Input: dimensioned drawing with shaded views. Units: mm. Origin: part minimum x, y, z. Give positions to 0.01 mm unless a question says otherwise; leave off trailing zeros. Write each loop counter-clockwise with the first axis right and the second up, starting at its lowest first coordinate (ties: lowest second). Pieces come first, ordered by that corner, then holes. Notation, with made-up numbers: (64.25, 4) -> (88.25, 4) arc R19 cw to (88.25, 38) -> close; hole circle Ø2 at (87.5, 50.5). An arc over 180 degrees is marked (long way). Answer as a JSON object with one key per item and string values.
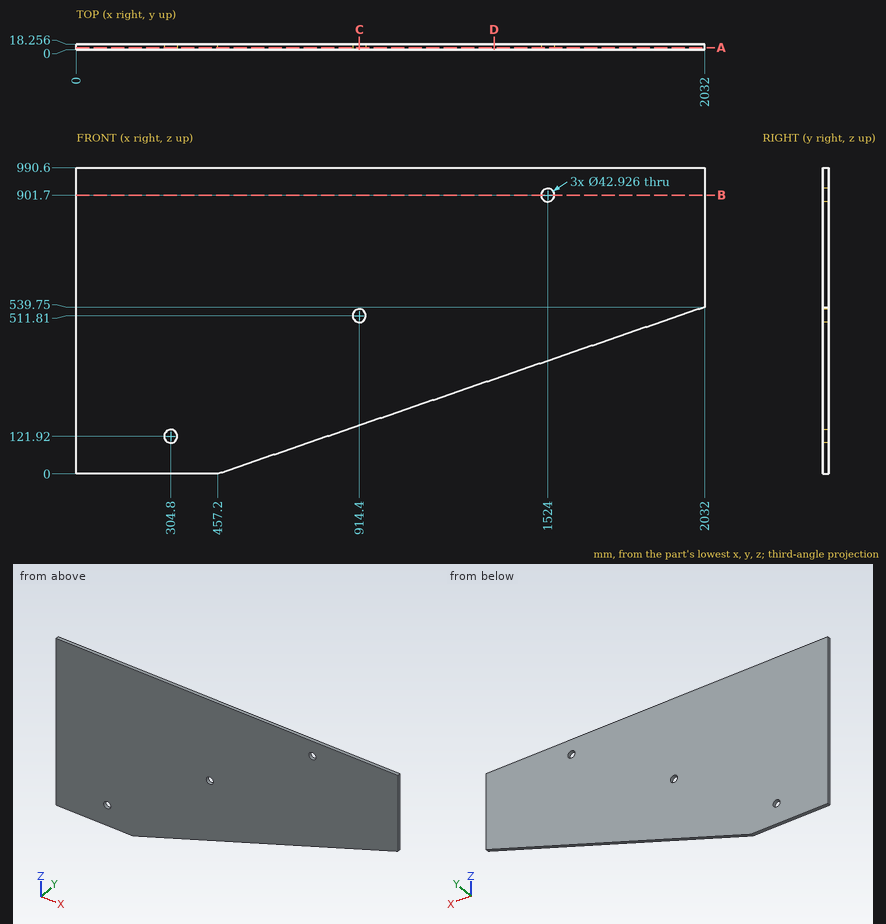
Q1. Cut plane B-B (z = 901.7). Return the cut outline in (x, y).
Values:
{"outline": "(0, 0) -> (1502.54, 0) -> (1502.54, 18.26) -> (0, 18.26) -> close; (1545.46, 0) -> (2032, 0) -> (2032, 18.26) -> (1545.46, 18.26) -> close"}
Q2. Cut plane D-D (x = 1350.5). Return the cut outline in (y, z).
Values:
{"outline": "(0, 306.17) -> (18.26, 306.17) -> (18.26, 990.6) -> (0, 990.6) -> close"}
Q3. Cut plane C-C (x = 914.4). Return the cut outline in (y, z).
Values:
{"outline": "(0, 156.7) -> (18.26, 156.7) -> (18.26, 490.35) -> (0, 490.35) -> close; (0, 533.27) -> (18.26, 533.27) -> (18.26, 990.6) -> (0, 990.6) -> close"}
Q4. First-contact query: P1, Ø5, axis at x = 1262.5, y = 14, coming from the -Z side; P2, Ø10, axis at x = 1666.5, y = 13, coming from the -Z side. Flat tips, straight axial feed; report the tip coordinate or a pass-through.
Values:
{"P1": "z = 275.15", "P2": "z = 412.76"}
Q5. Cut plane A-A (y = 6.75). Return the cut outline in (x, z), and give its area (3 significant figures).
Values:
{"outline": "(0, 0) -> (457.2, 0) -> (2032, 539.75) -> (2032, 990.6) -> (0, 990.6) -> close; hole circle Ø42.93 at (304.8, 121.92); hole circle Ø42.93 at (914.4, 511.81); hole circle Ø42.93 at (1524, 901.7)", "area": "1,580,000 mm²"}
Q6. Material intervals for L1, parallel to Z at x = 304.8, y = 7; L2, parallel to Z at x = 914.4, y = 11.75; L3, parallel to Z at x = 745.5, y = 11.25, sorted ascending. Write a range as from..to.
Values:
{"L1": "0..100.46, 143.38..990.6", "L2": "156.7..490.35, 533.27..990.6", "L3": "98.81..990.6"}
